from build123d import *

# Parameters (mm, degrees)
F1_W      = 30
F1_H      = 35
F2_DEPTH  = 10
F3_W      = 23
F3_H      = 9
F4_DEPTH  = 3
F6_DEPTH  = 8
F7_W      = 9
F7_H      = 10
F8_DEPTH  = 8
F9_W      = 5.75
F9_H      = 1.9
F9_W_2    = 5.5
F10_DEPTH = 3
F11_W     = 6.5
F11_H     = 5
F12_DEPTH = 3
F13_W     = 6.5
F13_H     = 5
F14_DEPTH = 3


with BuildPart() as f2:
    # F1 (on face) → F2 (new body)
    with BuildSketch(Plane.XY):
        Rectangle(F1_W, F1_H)
    extrude(amount=F2_DEPTH)

    # F3 (on face) → F4 (cut)
    with BuildSketch(Plane.XY):
        Rectangle(F3_W, F3_H)
    extrude(amount=F4_DEPTH, mode=Mode.SUBTRACT)

    # F5 (on face) → F6 (cut)
    with BuildSketch(Plane.XY):
        Polygon((-5.5, 14), (-5.5, 6), (5.5, 6), (5.5, 14), (4.75, 15), (-4.75, 15), align=None)
    extrude(amount=F6_DEPTH, mode=Mode.SUBTRACT)

    # F7 (on face) → F8 (cut)
    with BuildSketch(Plane.XY):
        with Locations((0, -11)):
            Rectangle(F7_W, F7_H)
    extrude(amount=F8_DEPTH, mode=Mode.SUBTRACT)

    # F9 (on face) → F10 (join, through all)
    with BuildSketch(Plane(origin=(0, 0, 3), x_dir=(1, 0, 0), z_dir=(0, 0, -1))):
        with Locations((6.975, 1.8)):
            Rectangle(F9_W, F9_H)
        with Locations((-7.1, -1.8)):
            Rectangle(F9_W_2, F9_H)
        with Locations((1.225, 1.8)):
            Rectangle(F9_W, F9_H)
    extrude(amount=F10_DEPTH)

    # F11 (on face) → F12 (cut)
    with BuildSketch(Plane(origin=(0, 6, 0), x_dir=(-1, 0, 0), z_dir=(0, 1, 0))):
        with Locations((0, 5.5)):
            Rectangle(F11_W, F11_H)
    extrude(amount=-F12_DEPTH, mode=Mode.SUBTRACT)

    # F13 (on face) → F14 (cut)
    with BuildSketch(Plane.XZ.offset(6)):
        with Locations((0, 5.5)):
            Rectangle(F13_W, F13_H)
    extrude(amount=-F14_DEPTH, mode=Mode.SUBTRACT)


solid = f2.part
Design review of the part built by this model. Coordinates are the model's own, in mm. A direction names the side the tool comes from. Give positions to 0.01 mm unless a question says otherwise; leave off trailing zeros. Write each loop counter-clockwise with the first axis right and the second up, starting at its lowest first coordinate (ties: lowest second). Pieces come first, ordered by that corner, then holes. Notation, with made-up numbers: M 1,-40 L 44,-40 A12 cw 44,-27 Z; hole C -20,-11.5 d11. An arc over 180 degrees is marked long. Answer as a JSON object with one key per item and string values. Group by question number.
1) Tool access review of faces 5 (the face through (4, -2.75, 2)), 6 (the face through (3.25, 5, 5)): name each direction out of +Z, -Z, +X, -X, +Y, -Y from which nothing blocks a thin tool from reaching the whole face with its end or side.
2) We need section C-C (y = -11). Give the boundary of the cut face in (x, z), and give its area (3 significant figures).
3) We need section A-A (z = 1.75). Give the boundary of the cut face in (x, y), and give its area (3 significant figures).
4) For line 1 along Y through (x, z) = (1.25, 0.5); line 2 along X through (y, z) = (-2, 1.75); line 3 along X through (y, z) = (11, 1.5), list the stretches that pass through material, from the lowest coordinate up.
5) We need section B-B (x = -2.5). Give the boundary of the cut face in (y, z).
6) We need section D-D (x = -10.25). Give the boundary of the cut face in (y, z).
7) Mouldability with a two-part tool opening along Y and no side actions: class faces 1 (the face through (0, 17.5, 5)), 2 (the face through (-15, 0, 5)), 3 (the face through (11.5, 0, 1)), 4 (the face through (0, -17.5, 5)) as released by +Y, released by -Y, zero draft, split by the parting line, or undercut.
Answer key:
{
 "1": {"face 5": "-Z", "face 6": "none"},
 "2": {"outline": "M -15,0 L -4.5,0 L -4.5,8 L 4.5,8 L 4.5,0 L 15,0 L 15,10 L -15,10 Z", "area": "228 mm²"},
 "3": {"outline": "M -15,-17.5 L 15,-17.5 L 15,17.5 L -15,17.5 Z; M -9.85,0.85 L -4.35,0.85 L -4.35,2.75 L -9.85,2.75 Z; M -1.65,-2.75 L 9.85,-2.75 L 9.85,-0.85 L -1.65,-0.85 Z; hole M -11.5,-4.5 L 11.5,-4.5 L 11.5,4.5 L -11.5,4.5 Z; hole M -5.5,6 L 5.5,6 L 5.5,14 L 4.75,15 L -4.75,15 L -5.5,14 Z; hole M -4.5,-16 L 4.5,-16 L 4.5,-6 L -4.5,-6 Z", "area": "687 mm²"},
 "4": {"line 1": "y = -17.5 to -16, -6 to -4.5, -2.75 to -0.85, 4.5 to 6, 15 to 17.5", "line 2": "x = -15 to -11.5, -1.65 to 9.85, 11.5 to 15", "line 3": "x = -15 to -5.5, 5.5 to 15"},
 "5": {"outline": "M -17.5,0 L -16,0 L -16,8 L -3,8 L -3,3 L 3,3 L 3,8 L 15,8 L 15,0 L 17.5,0 L 17.5,10 L -17.5,10 Z; M -6,0 L -4.5,0 L -4.5,3 L -6,3 Z; M 4.5,0 L 6,0 L 6,3 L 4.5,3 Z"},
 "6": {"outline": "M -17.5,0 L -4.5,0 L -4.5,3 L 4.5,3 L 4.5,0 L 17.5,0 L 17.5,10 L -17.5,10 Z"},
 "7": {"face 1": "released by +Y", "face 2": "zero draft", "face 3": "undercut", "face 4": "released by -Y"}
}
